from build123d import *

# Parameters (mm, degrees)
F0_W          = 32
F0_H          = 32
F0_R          = 1.9778790134
F0_R_2        = 2.1975244048
F0_R_3        = 1.8387533056
F0_R_4        = 6
F0_R_5        = 1.6790844608
F1_DEPTH      = 6
F2_R          = 10.5
F2_R_2        = 6
F3_DEPTH      = 24
F4_SIZE       = 2
F5_R          = 11.2136661157
F5_R_2        = 10.5
F6_DEPTH      = 1
F7_R          = 9.7938073019
F7_R_2        = 6.6264369037
F8_DEPTH      = 1
F9_SIZE       = 0.5
F10_R         = 8.3375339565
F10_R_2       = 6.4778965527
F11_DEPTH     = 1
F12_T1_DEPTH  = 30.571682988
F12_T3_DEPTH  = 5.4001101127
F12_T5_DEPTH  = 5.4001101127
F12_T7_DEPTH  = 30.571682988
F12_T9_DEPTH  = 5.4001101127
F12_T11_DEPTH = 5.4001101127


# Not quite as in the source:
# - a fillet or chamfer that OpenCascade refuses, or shapes differently, is made with other operations: its cross-section is extruded or revolved along the edge and cut away or added


with BuildPart() as f1:
    # F0 (on Top) → F1 (new body)
    with BuildSketch(Plane.XY):
        Rectangle(F0_W, F0_H)
        with Locations((-11.313708499, -11.313708499)):
            Circle(F0_R, mode=Mode.SUBTRACT)
        with Locations((11.313708499, -11.313708499)):
            Circle(F0_R_2, mode=Mode.SUBTRACT)
        with Locations((-11.313708499, 11.313708499)):
            Circle(F0_R_3, mode=Mode.SUBTRACT)
        Circle(F0_R_4, mode=Mode.SUBTRACT)
        with Locations((11.313708499, 11.313708499)):
            Circle(F0_R_5, mode=Mode.SUBTRACT)
    extrude(amount=F1_DEPTH)

    # F2 (on face) → F3 (join)
    with BuildSketch(Plane.XY.offset(6)):
        Circle(F2_R)
        Circle(F2_R_2, mode=Mode.SUBTRACT)
    extrude(amount=F3_DEPTH)

    # F4
    f4_edges = [f1.edges().sort_by_distance(p)[0] for p in [
        (-16, -16, 3),
        (16, -16, 3),
        (-16, 16, 3),
        (16, 16, 3),
    ]]
    chamfer(f4_edges, length=F4_SIZE)

    # F5 (on face) → F6 (cut)
    with BuildSketch(Plane.XY.offset(6)):
        Circle(F5_R)
        Circle(F5_R_2, mode=Mode.SUBTRACT)
    extrude(amount=-F6_DEPTH, mode=Mode.SUBTRACT)

    # F7 (on face) → F8 (cut)
    with BuildSketch(Plane.XY.offset(30)):
        Circle(F7_R)
        Circle(F7_R_2, mode=Mode.SUBTRACT)
    extrude(amount=-F8_DEPTH, mode=Mode.SUBTRACT)

    # F9
    f9_edges = [f1.edges().sort_by_distance(p)[0] for p in [
        (-13.291588, -11.313708, 6),
        (9.634624, 11.313708, 6),
        (9.116184, -11.313708, 6),
        (-13.152462, 11.313708, 6),
    ]]
    chamfer(f9_edges, length=F9_SIZE)

    # F10 (on face) → F11 (cut)
    with BuildSketch(Plane(origin=(0, 0, 0), x_dir=(1, 0, 0), z_dir=(0, 0, -1))):
        Circle(F10_R)
        Circle(F10_R_2, mode=Mode.SUBTRACT)
    extrude(amount=-F11_DEPTH, mode=Mode.SUBTRACT)

    # F12: chamfer of 0.5 on 26 edges, made by hand

    # F12_s2 → F12_t1 (cut)
    with BuildSketch(Plane.YZ.offset(-15.285841494)):
        Polygon((-16, 0.5), (-15.5, 0), (-16, 0), align=None)
        Polygon((16, 0.5), (15.5, 0), (16, 0), align=None)
        Polygon((-15.5, 6), (-16, 5.5), (-16, 6), align=None)
        Polygon((15.5, 6), (16, 5.5), (16, 6), align=None)
    extrude(amount=F12_T1_DEPTH, mode=Mode.SUBTRACT)

    # F12_s4 → F12_t3 (cut)
    with BuildSketch(Plane(origin=(1.9092272399, -1.9092272399, 0), x_dir=(0, 0, 1), z_dir=(-0.7071067812, 0.7071067812, 0))):
        Polygon((0.5, -21.2132034356), (0, -20.7132034356), (0, -21.2132034356), align=None)
        Polygon((6, -20.7132034356), (5.5, -21.2132034356), (6, -21.2132034356), align=None)
    extrude(amount=F12_T3_DEPTH, mode=Mode.SUBTRACT)

    # F12_s6 → F12_t5 (cut)
    with BuildSketch(Plane(origin=(-1.9092272399, -1.9092272399, 0), x_dir=(0, 0, 1), z_dir=(0.7071067812, 0.7071067812, 0))):
        Polygon((0.5, 21.2132034356), (0, 20.7132034356), (0, 21.2132034356), align=None)
        Polygon((6, 20.7132034356), (5.5, 21.2132034356), (6, 21.2132034356), align=None)
    extrude(amount=F12_T5_DEPTH, mode=Mode.SUBTRACT)

    # F12_s8 → F12_t7 (cut)
    with BuildSketch(Plane.XZ.offset(-15.285841494)):
        Polygon((-16, 0.5), (-15.5, 0), (-16, 0), align=None)
        Polygon((16, 0.5), (15.5, 0), (16, 0), align=None)
        Polygon((-15.5, 6), (-16, 5.5), (-16, 6), align=None)
        Polygon((15.5, 6), (16, 5.5), (16, 6), align=None)
    extrude(amount=F12_T7_DEPTH, mode=Mode.SUBTRACT)

    # F12_s10 → F12_t9 (cut)
    with BuildSketch(Plane(origin=(1.9092272399, 1.9092272399, 0), x_dir=(0, 0, 1), z_dir=(-0.7071067812, -0.7071067812, 0))):
        Polygon((0.5, 21.2132034356), (0, 20.7132034356), (0, 21.2132034356), align=None)
        Polygon((6, 20.7132034356), (5.5, 21.2132034356), (6, 21.2132034356), align=None)
    extrude(amount=F12_T9_DEPTH, mode=Mode.SUBTRACT)

    # F12_s12 → F12_t11 (cut)
    with BuildSketch(Plane(origin=(-1.9092272399, 1.9092272399, 0), x_dir=(0, 0, 1), z_dir=(0.7071067812, -0.7071067812, 0))):
        Polygon((0.5, -21.2132034356), (0, -20.7132034356), (0, -21.2132034356), align=None)
        Polygon((6, -20.7132034356), (5.5, -21.2132034356), (6, -21.2132034356), align=None)
    extrude(amount=F12_T11_DEPTH, mode=Mode.SUBTRACT)

    # F12_s13 → F12_t14 (revolve, cut)
    with BuildSketch(Plane.XZ.offset(11.313708499)):
        Polygon((-9.3358294856, 0.5), (-8.8358294856, 0), (-9.3358294856, 0), align=None)
    revolve(axis=Axis((-11.313708499, -11.313708499, 0), (0, 0, 1)), mode=Mode.SUBTRACT)

    # F12_s15 → F12_t16 (revolve, cut)
    with BuildSketch(Plane.XZ.offset(11.313708499)):
        Polygon((14.0112329038, 0), (13.5112329038, 0.5), (13.5112329038, 0), align=None)
    revolve(axis=Axis((11.313708499, -11.313708499, 0), (0, 0, 1)), mode=Mode.SUBTRACT)

    # F12_s17 → F12_t18 (revolve, cut)
    with BuildSketch(Plane.XZ):
        Polygon((8.8375339565, 0), (8.3375339565, 0.5), (8.3375339565, 0), align=None)
    revolve(axis=Axis((0, 0, 0), (0, 0, -1)), mode=Mode.SUBTRACT)

    # F12_s19 → F12_t20 (revolve, cut)
    with BuildSketch(Plane.XZ.offset(-11.313708499)):
        Polygon((-8.9749551934, 0), (-9.4749551934, 0.5), (-9.4749551934, 0), align=None)
    revolve(axis=Axis((-11.313708499, 11.313708499, 0), (0, 0, 1)), mode=Mode.SUBTRACT)

    # F12_s21 → F12_t22 (revolve, cut)
    with BuildSketch(Plane.XZ.offset(-11.313708499)):
        Polygon((13.4927929597, 0), (12.9927929597, 0.5), (12.9927929597, 0), align=None)
    revolve(axis=Axis((11.313708499, 11.313708499, 0), (0, 0, 1)), mode=Mode.SUBTRACT)

    # F12_s23 → F12_t24 (revolve, cut)
    with BuildSketch(Plane.XZ.offset(11.313708499)):
        Polygon((-8.6287227044, 6), (-8.982276095, 5.8535533906), (-8.8358294856, 6), align=None)
    revolve(axis=Axis((-11.313708499, -11.313708499, 6), (0, 0, 1)), mode=Mode.SUBTRACT)

    # F12_s25 → F12_t26 (revolve, cut)
    with BuildSketch(Plane.XZ):
        Polygon((11.7136661157, 6), (11.2136661157, 5.5), (11.2136661157, 6), align=None)
    revolve(axis=Axis((0, 0, 6), (0, 0, 1)), mode=Mode.SUBTRACT)

    # F12_s27 → F12_t28 (revolve, cut)
    with BuildSketch(Plane.XZ.offset(-11.313708499)):
        Polygon((13.6998997409, 6), (13.3463463503, 5.8535533906), (13.4927929597, 6), align=None)
    revolve(axis=Axis((11.313708499, 11.313708499, 6), (0, 0, 1)), mode=Mode.SUBTRACT)

    # F12_s29 → F12_t30 (revolve, cut)
    with BuildSketch(Plane.XZ.offset(11.313708499)):
        Polygon((14.218339685, 6), (13.8647862944, 5.8535533906), (14.0112329038, 6), align=None)
    revolve(axis=Axis((11.313708499, -11.313708499, 6), (0, 0, 1)), mode=Mode.SUBTRACT)

    # F12_s31 → F12_t32 (revolve, cut)
    with BuildSketch(Plane.XZ.offset(-11.313708499)):
        Polygon((-8.7678484122, 6), (-9.1214018028, 5.8535533906), (-8.9749551934, 6), align=None)
    revolve(axis=Axis((-11.313708499, 11.313708499, 6), (0, 0, 1)), mode=Mode.SUBTRACT)


solid = f1.part
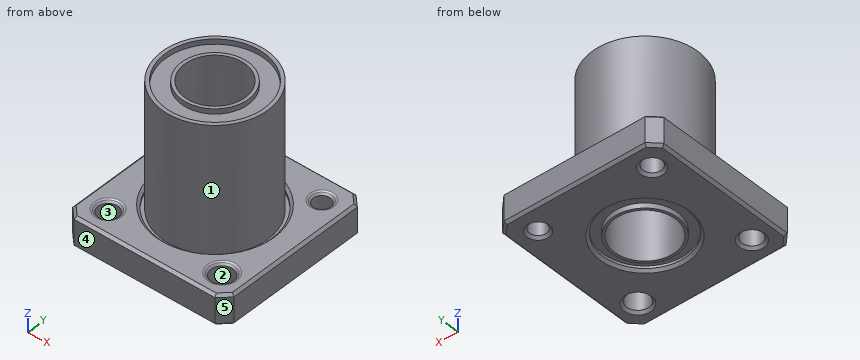
Model file for the job. Use its own axes, mm. Face numbers are marked on the shaded views. A direction names the side the tool comes from. Coordinates: 2 decimals unless noted, no trailing zeros. Order: outer loops, then holes, each group sorted by start corner. A loop starts at its lowest first (then second) coordinate and runs counter-clockwise, first axis right, second up. Notation, with made-up numbers: (-21, 7) -> (-3, 7) arc R25 cw to (-3, 42) -> close; hole circle Ø9 at (-29, 34.5). An arc over 180 degrees is marked (long way). Return JSON: item names as keys, results as strings. Group by question number.
Item 1: Saw through at A-A on z = 13. Write the cut outline in (x, y), then the cut area to 3 significant figures.
Item 2: Pull direction X, two halves, no side cores. Call the marked faces 3, 4 and 5: pulls with the +X half, pulls with the -X half, needs draft (parallel to the pull), parting line crosses it, or undercut.
Item 3: Wall check: line 1 along Y through (x, z) = (0, 0.7); line 2 along Y through (x, z) = (0, 5.4); line 3 along Y through (x, z) = (-11, 2.5). Give the ranges that are in metal, low to high. Write a range as [from, to].
Item 4: Tool access for the marked faces 1 and 2: list every direction of +Z, -Z, +X, -X, +Y, -Y with a clear straight run to the whole face (end or side of a thin tool).
Item 5: Flat gauge pins, fed straight in: P1, Ø2, axis at y = -6, z = 8, coming from the -X side; P2, Ø2, axis at x = -10, z = 23, coming from the +Y side; P3, Ø1.5, axis at y = -4, z = 9, coming from the -X side; P4, Ø13.5, axis at x = 2, y = 3.5, coming from the -Z side. Where does each tip first touch, or does it go through?
Values found:
{
 "1": {"outline": "circle Ø21 at (0, 0); hole circle Ø12 at (0, 0)", "area": "233 mm2"},
 "2": {"face 3": "undercut", "face 4": "needs draft", "face 5": "pulls with the +X half"},
 "3": {"line 1": "y = [-16, -8.34], [-6.48, -6], [6, 6.48], [8.34, 16]", "line 2": "y = [-16, -11.21], [-10.5, -6], [6, 10.5], [11.21, 16]", "line 3": "y = [-16, -13.27], [-9.36, 9.5], [13.13, 16]"},
 "4": {"face 1": "+Z", "face 2": "+Z, -Z"},
 "5": {"P1": "stops at x = -9.23", "P2": "stops at y = 5.41", "P3": "stops at x = -9.98", "P4": "stops at z = 0"}
}
